The model under review builds one solid part; all positions refer to its coordinate system, in mm. Face numbers are marked on the shaded views. A direction names the side the tool comes from. Coordinates: 2 decimals unless noted, no trailing zeros. Write each loop counter-clockwise with the first axis right and the second up, starting at its lowest first coordinate (ties: lowest second). Pieces come first, ordered by that corner, then holes. Notation, with made-up numbers: (-26.5, -20) - (-17.5, -20) arc R27 ccw to (-17.5, 13) - close; hole circle Ø8 at (52.5, 30). An arc over 180 degrees is marked (long way). Return JSON: item names as keys, results as strings. Group by question number.
(1) For pin 1 Ø5 at (x, z) = (11, 30.5) entering from +Y; pin 2 Ø6 at (x, y) = (-5.5, -4.5) entering from +Z; pin 3 Ø5 at (x, z) = (10.5, 41) entering from -Y, all flat-tipped, find the tip position at first contact; note any pin that passes through.
(2) We need section C-C on x = -2. Give the number of separate pieces and of enclosed holes in the cut face, then the cut area to 3 significant figures.
(3) Draft analysis for pull direction Y (two halves, no side actions). For the marked faces 1, 2 and 3, state which applies: released by +Y, released by -Y, zero draft, split by the parting line, or undercut.
(4) We need section D-D on x = 10. State the section outline as (y, z) points, then the cut area to 3 significant figures.
(5) To check wall thickness, follow L1, parallel to Y at x = 0, z = 56; L2, parallel to Y at x = -1.5, z = 59.5; L3, parallel to Y at x = -12.5, z = 50. State the ranges of each line that lie inside material, in increasing order. Write a range as from..to.
(6) We need section B-B on z = 50.5. State the section outline as (x, y) points.
(7) Tool access review of the marked faces 4 and 5: name each direction out of +Z, -Z, +X, -X, +Y, -Y from which nothing blocks a thin tool from reaching the whole face with its end or side.
(8) We need section A-A on y = 0. State the section outline as (x, z) points, then the cut area to 3 significant figures.
```python
from build123d import *

# Parameters (mm, degrees)
SKETCH2_R              = 15
SKETCH2_R_2            = 13.5
SKETCH2_R_3            = 3
SHELL_DEPTH            = 80
SKETCH8_R              = 2.75
INNERPARTITION_DEPTH   = 2.5
MOVE_START             = 40
MOVE_FACE6_OUTLINE_R   = 2.75
MOVE_FACE6_DEPTH       = 2.5
MOVE_START_2           = 55
MOVE_FACE6_2_OUTLINE_R = 2.75
MOVE_FACE6_2_DEPTH     = 2.5
EASIER_ASSEMBLY_DEPTH  = 5


# Read off the part's stored shape, not the designer's step: Move Face6
with BuildPart() as part:
    # Sketch2 → Shell (new body)
    # profile 1 of 6: a face of its own
    with BuildSketch(Plane.XY):
        Circle(SKETCH2_R)
        Circle(SKETCH2_R_2, mode=Mode.SUBTRACT)
    # profile 2 of 6: a face of its own
    with BuildSketch(Plane.XY):
        with BuildLine():
            ThreePointArc((-2.727178029, 14.75), (-2.962055082, 13.975636094), (-2.98142397, 13.166666667))
            ThreePointArc((-2.98142397, 13.166666667), (0, 13.5), (2.98142397, 13.166666667))
            ThreePointArc((2.98142397, 13.166666667), (2.962055082, 13.975636094), (2.727178029, 14.75))
            ThreePointArc((2.727178029, 14.75), (0, 15), (-2.727178029, 14.75))
        make_face()
    # profile 3 of 6: a face of its own
    with BuildSketch(Plane.XY):
        with BuildLine():
            ThreePointArc((-13.452587926, -1.130432705), (-13.5, 0), (-13.452587926, 1.130432705))
            ThreePointArc((-13.452587926, 1.130432705), (-10.18513224, 8.860760761), (-2.98142397, 13.166666667))
            ThreePointArc((-2.98142397, 13.166666667), (-2.962055082, 13.975636094), (-2.727178029, 14.75))
            ThreePointArc((-2.727178029, 14.75), (-15, 0), (-2.727178029, -14.75))
            ThreePointArc((-2.727178029, -14.75), (-2.962055082, -13.975636094), (-2.98142397, -13.166666667))
            ThreePointArc((-2.98142397, -13.166666667), (-10.18513224, -8.860760761), (-13.452587926, -1.130432705))
        make_face()
    # profile 4 of 6: a face of its own
    with BuildSketch(Plane.XY):
        with BuildLine():
            ThreePointArc((2.727178029, 14.75), (2.962055082, 13.975636094), (2.98142397, 13.166666667))
            ThreePointArc((2.98142397, 13.166666667), (10.18513224, 8.860760761), (13.452587926, 1.130432705))
            ThreePointArc((13.452587926, 1.130432705), (13.488141773, 0.565713268), (13.5, 0))
            ThreePointArc((13.5, 0), (13.488141773, -0.565713268), (13.452587926, -1.130432705))
            ThreePointArc((13.452587926, -1.130432705), (10.18513224, -8.860760761), (2.98142397, -13.166666667))
            ThreePointArc((2.98142397, -13.166666667), (2.962055082, -13.975636094), (2.727178029, -14.75))
            ThreePointArc((2.727178029, -14.75), (11.530560924, -9.594069251), (15, 0))
            ThreePointArc((15, 0), (11.530560924, 9.594069251), (2.727178029, 14.75))
        make_face()
    # profile 5 of 6: a face of its own
    with BuildSketch(Plane.XY):
        with BuildLine():
            ThreePointArc((2.98142397, -13.166666667), (0, -13.5), (-2.98142397, -13.166666667))
            ThreePointArc((-2.98142397, -13.166666667), (-2.962055082, -13.975636094), (-2.727178029, -14.75))
            ThreePointArc((-2.727178029, -14.75), (0, -15), (2.727178029, -14.75))
            ThreePointArc((2.727178029, -14.75), (2.962055082, -13.975636094), (2.98142397, -13.166666667))
        make_face()
    # profile 6 of 6: a face of its own
    with BuildSketch(Plane.XY):
        with BuildLine():
            Line((-3.312419342, 1.130432705), (-13.452587926, 1.130432705))
            ThreePointArc((-13.452587926, 1.130432705), (-13.5, 0), (-13.452587926, -1.130432705))
            Line((-13.452587926, -1.130432705), (-3.312419342, -1.130432705))
            ThreePointArc((-3.312419342, -1.130432705), (0, -3.5), (3.312419342, -1.130432705))
            Line((3.312419342, -1.130432705), (13.452587926, -1.130432705))
            ThreePointArc((13.452587926, -1.130432705), (13.488141773, -0.565713268), (13.5, 0))
            ThreePointArc((13.5, 0), (13.488141773, 0.565713268), (13.452587926, 1.130432705))
            Line((13.452587926, 1.130432705), (3.312419342, 1.130432705))
            ThreePointArc((3.312419342, 1.130432705), (0, 3.5), (-3.312419342, 1.130432705))
        make_face()
        Circle(SKETCH2_R_3, mode=Mode.SUBTRACT)
    extrude(amount=SHELL_DEPTH)

    # Sketch8 → InnerPartition (add)
    # profile 1 of 2: a face of its own
    with BuildSketch(Plane.XY.offset(40)):
        with BuildLine():
            ThreePointArc((13.452587926, 1.130432705), (0, 13.5), (-13.452587926, 1.130432705))
            Line((-13.452587926, 1.130432705), (-3.312419342, 1.130432705))
            ThreePointArc((-3.312419342, 1.130432705), (0, 3.5), (3.312419342, 1.130432705))
            Line((3.312419342, 1.130432705), (13.452587926, 1.130432705))
        make_face()
        with Locations((0, 8)):
            Circle(SKETCH8_R, mode=Mode.SUBTRACT)
    # profile 2 of 2: a face of its own
    with BuildSketch(Plane.XY.offset(40)):
        with BuildLine():
            Line((-3.312419342, -1.130432705), (-13.452587926, -1.130432705))
            ThreePointArc((-13.452587926, -1.130432705), (0, -13.5), (13.452587926, -1.130432705))
            Line((13.452587926, -1.130432705), (3.312419342, -1.130432705))
            ThreePointArc((3.312419342, -1.130432705), (0, -3.5), (-3.312419342, -1.130432705))
        make_face()
        with Locations((0, -8)):
            Circle(SKETCH8_R, mode=Mode.SUBTRACT)
    extrude(amount=INNERPARTITION_DEPTH)

    # Move Face6 outline → Move Face6 (cut)
    # profile 1 of 2: a face of its own
    with BuildSketch(Plane.XY.offset(MOVE_START)):
        with BuildLine():
            ThreePointArc((-13.452587926, -1.130432705), (0, -13.5), (13.452587926, -1.130432705))
            Line((13.452587926, -1.130432705), (3.312419342, -1.130432705))
            ThreePointArc((3.312419342, -1.130432705), (0, -3.5), (-3.312419342, -1.130432705))
            Line((-3.312419342, -1.130432705), (-13.452587926, -1.130432705))
        make_face()
        with Locations((0, -8)):
            Circle(MOVE_FACE6_OUTLINE_R, mode=Mode.SUBTRACT)
    # profile 2 of 2: a face of its own
    with BuildSketch(Plane.XY.offset(MOVE_START)):
        with BuildLine():
            ThreePointArc((13.452587926, 1.130432705), (0, 13.5), (-13.452587926, 1.130432705))
            Line((-13.452587926, 1.130432705), (-3.312419342, 1.130432705))
            ThreePointArc((-3.312419342, 1.130432705), (0, 3.5), (3.312419342, 1.130432705))
            Line((3.312419342, 1.130432705), (13.452587926, 1.130432705))
        make_face()
        with Locations((0, 8)):
            Circle(MOVE_FACE6_OUTLINE_R, mode=Mode.SUBTRACT)
    extrude(amount=MOVE_FACE6_DEPTH, mode=Mode.SUBTRACT)

    # Move Face6 2 outline → Move Face6 2 (add)
    # profile 1 of 2: a face of its own
    with BuildSketch(Plane.XY.offset(MOVE_START_2)):
        with BuildLine():
            ThreePointArc((-13.452587926, -1.130432705), (0, -13.5), (13.452587926, -1.130432705))
            Line((13.452587926, -1.130432705), (3.312419342, -1.130432705))
            ThreePointArc((3.312419342, -1.130432705), (0, -3.5), (-3.312419342, -1.130432705))
            Line((-3.312419342, -1.130432705), (-13.452587926, -1.130432705))
        make_face()
        with Locations((0, -8)):
            Circle(MOVE_FACE6_2_OUTLINE_R, mode=Mode.SUBTRACT)
    # profile 2 of 2: a face of its own
    with BuildSketch(Plane.XY.offset(MOVE_START_2)):
        with BuildLine():
            ThreePointArc((13.452587926, 1.130432705), (0, 13.5), (-13.452587926, 1.130432705))
            Line((-13.452587926, 1.130432705), (-3.312419342, 1.130432705))
            ThreePointArc((-3.312419342, 1.130432705), (0, 3.5), (3.312419342, 1.130432705))
            Line((3.312419342, 1.130432705), (13.452587926, 1.130432705))
        make_face()
        with Locations((0, 8)):
            Circle(MOVE_FACE6_2_OUTLINE_R, mode=Mode.SUBTRACT)
    extrude(amount=MOVE_FACE6_2_DEPTH)

    # Sketch2<12> → Easier assembly (cut)
    with BuildSketch(Plane.XY):
        with BuildLine():
            ThreePointArc((-2.727178029, 14.75), (-2.962055082, 13.975636094), (-2.98142397, 13.166666667))
            ThreePointArc((-2.98142397, 13.166666667), (0, 13.5), (2.98142397, 13.166666667))
            ThreePointArc((2.98142397, 13.166666667), (2.962055082, 13.975636094), (2.727178029, 14.75))
            ThreePointArc((2.727178029, 14.75), (0, 15), (-2.727178029, 14.75))
        make_face()
        with BuildLine():
            ThreePointArc((2.98142397, -13.166666667), (0, -13.5), (-2.98142397, -13.166666667))
            ThreePointArc((-2.98142397, -13.166666667), (-2.962055082, -13.975636094), (-2.727178029, -14.75))
            ThreePointArc((-2.727178029, -14.75), (0, -15), (2.727178029, -14.75))
            ThreePointArc((2.727178029, -14.75), (2.962055082, -13.975636094), (2.98142397, -13.166666667))
        make_face()
    extrude(amount=EASIER_ASSEMBLY_DEPTH, mode=Mode.SUBTRACT)


solid = part.part
```
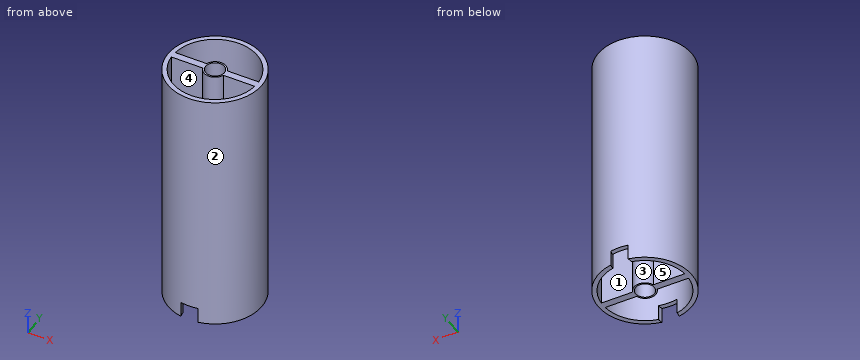
Ans:
{
 "1": {"pin 1": "y = 12.36", "pin 2": "z = 57.5", "pin 3": "y = -12.69"},
 "2": {"separate pieces": "4", "enclosed holes": "0", "area": "363 mm²"},
 "3": {"face 1": "undercut", "face 2": "split by the parting line", "face 3": "undercut"},
 "4": {"outline": "(-11.18, 0) - (-9.07, 0) - (-9.07, 55) - (-1.13, 55) - (-1.13, 0) - (1.13, 0) - (1.13, 55) - (9.07, 55) - (9.07, 0) - (11.18, 0) - (11.18, 80) - (9.07, 80) - (9.07, 57.5) - (1.13, 57.5) - (1.13, 80) - (-1.13, 80) - (-1.13, 57.5) - (-9.07, 57.5) - (-9.07, 80) - (-11.18, 80) - close", "area": "558 mm²"},
 "5": {"L1": "-15..-10.75, -5.25..-3, 3..5.25, 10.75..15", "L2": "-14.92..-13.42, -3.16..-2.6, 2.6..3.16, 13.42..14.92", "L3": "-8.29..-5.1, -1.13..1.13, 5.1..8.29"},
 "6": {"outline": "circle Ø30 at (0, 0); hole (-13.45, -1.13) arc R13.5 ccw to (13.45, -1.13) - (3.31, -1.13) arc R3.5 cw to (-3.31, -1.13) - close; hole (-13.45, 1.13) - (-3.31, 1.13) arc R3.5 cw to (3.31, 1.13) - (13.45, 1.13) arc R13.5 ccw to start; hole circle Ø6 at (0, 0)"},
 "7": {"face 4": "+Z", "face 5": "-Z"},
 "8": {"outline": "(-15, 0) - (-3, 0) - (-3, 80) - (-15, 80) - close; (3, 0) - (15, 0) - (15, 80) - (3, 80) - close", "area": "1,920 mm²"}
}
